Check sheet for the modelled part. Datum: model origin and axes. Units: mm. Face numbers are marked on the shaded views. A direction names the side the tool comes from. Coordinates: 2 decimals unless noted, no trailing zeros. Loops run counter-clockwise (first coordinate to the right, second up) from the corner with the lowest first, then second, coordinate; pieces in that order, holes last. Notation, with made-up numbers: (45, 19) -> (91, 19) arc R16 ccw to (91, 32) -> close; hole circle Ø11 at (72.25, -8). An arc over 180 degrees is marked (long way). Use one line per item in the form item = value.
from build123d import *

# Parameters (mm, degrees)
F0_W     = 101.6
F0_H     = 25.4
F1_DEPTH = 152.4
F2_W     = 54.442895
F2_H     = 25.4
F3_DEPTH = 50.8
F5_DEPTH = 50.8


with BuildPart() as f1:
    # F0 (on Right) → F1 (new body)
    with BuildSketch(Plane.YZ):
        with Locations((10.159998, 4.812631)):
            Rectangle(F0_W, F0_H)
        Polygon((10.159998, 55.612631), (-40.640002, 17.512631), (60.959998, 17.512631), align=None)
    extrude(amount=-F1_DEPTH)

    # F2 (on face) → F3 (join)
    with BuildSketch(Plane.YZ):
        Polygon((9.17408, 37.297897), (-18.047368, 17.512631), (36.395527, 17.512631), align=None)
        with Locations((9.17408, 4.812631)):
            Rectangle(F2_W, F2_H)
    extrude(amount=F3_DEPTH)

    # F4 (on face) → F5 (join)
    with BuildSketch(Plane(origin=(0, 60.959998, 0), x_dir=(-1, 0, 0), z_dir=(0, 1, 0))):
        Polygon((63.967891, 55.612631), (33.287369, 17.512631), (103.137369, 17.512631), align=None)
    extrude(amount=-F5_DEPTH)


solid = f1.part
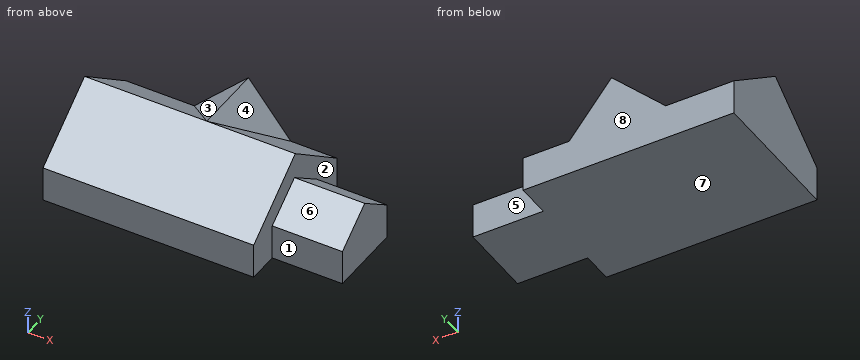
(1) Section check A-A, the plane z = 12. Record the boundary of the cut face in (x, y).
Established:
outline = (-152.4, -40.64) -> (0, -40.64) -> (0, -18.05) -> (50.8, -18.05) -> (50.8, 36.4) -> (0, 36.4) -> (0, 60.96) -> (-152.4, 60.96) -> close
(2) Scan lines: line 1 along X through (y, z) = (8, 46.5); line 2 along Y through (x, z) = (19, 5); line 3 along Y through (x, z) = (-67, 29). Record each from-to range of solid material in increasing order.
Established:
line_1 = -152.4 to 0
line_2 = -18.05 to 36.4
line_3 = -25.32 to 60.96
(3) Go/stop test with flat-tipped pins: P1, Ø6, axis at x = -101.5, y = -15.5, coming from the +Z side; P2, Ø8, axis at x = -115, z = 46.5, coming from the -Y side; P3, Ø20.5, axis at x = 18, z = 6.5, coming from the -Y side. Record where each tip stops, or that it passes through.
Established:
P1 = 38.62
P2 = -7.32
P3 = -18.05
(4) Section check D-D, the plane z = 43. Record the boundary of the cut face in (x, y), plus the area to 3 significant figures.
Established:
outline = (-152.4, -6.66) -> (0, -6.66) -> (0, 26.98) -> (-53.81, 26.98) -> (-53.81, 60.96) -> (-76.93, 60.96) -> (-76.93, 26.98) -> (-152.4, 26.98) -> close
area = 5,910 mm²
(5) Mould release check, pull along Z, two halves, no side actions. Record for the marked faces 6, 7 and 8: +Z half, -Z half, draft (parallel to the pull), parting line (faces both ways), or undercut.
Established:
face_6 = +Z half
face_7 = -Z half
face_8 = draft
(6) Section check B-B, the plane x = 11.5. Record the boundary of the cut face in (y, z).
Established:
outline = (-18.05, -7.89) -> (36.4, -7.89) -> (36.4, 17.51) -> (9.17, 37.3) -> (-18.05, 17.51) -> close
(7) Tool access check on the marked faces 1, 2, 3, 4 and 5. Record the directions out of +Z, -Z, +X, -X, +Y, -Y that give a thin tool (end or side, any length) a straight path to the whole face; none if there is none.
Established:
face_1 = +Z, -Z, +X, -Y
face_2 = +Z, +X
face_3 = +Z, -X, +Y
face_4 = +Z, +X, +Y
face_5 = +Z, -Z, +X, +Y
(8) Section check C-C, the plane y = 40. Record the boundary of the cut face in (x, z).
Established:
outline = (-152.4, -7.89) -> (0, -7.89) -> (0, 33.23) -> (-45.95, 33.23) -> (-63.97, 55.61) -> (-86.98, 33.23) -> (-152.4, 33.23) -> close
